Model file for the job. Use its own axes, mm. Give positions to 0.01 mm unless a question says otherwise; leave off trailing zeros. Write each loop counter-clockwise with the first axis right and the second up, starting at its lowest first coordinate (ties: lowest second). Pieces come first, ordered by that corner, then holes. Notation, with made-up numbers: (77, 78) - (93, 78) arc R17 cw to (93, 91) - close; hole circle Ø11 at (86, 54). An arc over 180 degrees is marked (long way). One line per item, written item: value. Start each with the question number.
(1) Cut at A-A, the plane y = 0. List the corners of the cut face in (x, z) (1 decimal), and give its area (3 significant figures).
(2) Cut at D-D, the plane x = 5. List the corners of the cut face in (y, z) (3 decimals), and give its area (3 significant figures).
(3) Probe L1, parallel to Y at x = 0, z = 1.2; L2, parallel to Y at x = 8, z = 1.7; L3, parallel to X at y = -14, z = 1.15. List the from-to ranges inside material, lowest first.
(4) Drop a flat-ended pin along its axis: P1, Ø1, axis at y = 10.5, z = 2, coming from the -X side. Give the stop position or say it passes through.
(5) Cut at C-C, the plane z = 1.3. List the corners of the cut face in (x, y) (1 decimal).
(6) Cut at B-B, the plane x = 0. List the corners of the cut face in (y, z) (3 decimals), and give its area (3 significant figures).
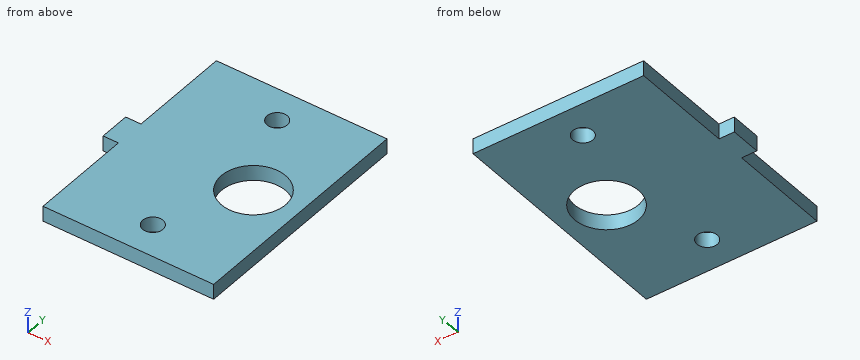
from build123d import *

# Parameters (mm, degrees)
SKETCH1_W           = 35.47213452
SKETCH1_H           = 48.789667988
BOSS_EXTRUDE1_DEPTH = 3.175
SKETCH2_R           = 2.10185
SKETCH2_R_2         = 6.6675
CUT_EXTRUDE1_DEPTH  = 31.327489716
BOSS_EXTRUDE2_DEPTH = 3.175


with BuildPart() as part:
    # Sketch1 → Boss-Extrude1 (new body)
    with BuildSketch(Plane.XY):
        Rectangle(SKETCH1_W, SKETCH1_H)
    extrude(amount=BOSS_EXTRUDE1_DEPTH)

    # Sketch2 → Cut-Extrude1 (cut, through all)
    with BuildSketch(Plane(origin=(0, 0, 0), x_dir=(-1, 0, 0), z_dir=(0, 0, -1))):
        with Locations((0, 17.5)):
            Circle(SKETCH2_R)
        with Locations((0, -17.5)):
            Circle(SKETCH2_R)
        with Locations((-8, 0)):
            Circle(SKETCH2_R_2)
    extrude(amount=-CUT_EXTRUDE1_DEPTH, mode=Mode.SUBTRACT)

    # Sketch3 → Boss-Extrude2 (add)
    with BuildSketch(Plane.ZY.offset(17.73606726)):
        Polygon((0, 0), (0, -3.175), (3.175, -3.175), (3.175, 3.175), (0, 3.175), align=None)
    extrude(amount=BOSS_EXTRUDE2_DEPTH)


solid = part.part
Answers follow:
1. outline: (-20.9, 0) - (1.3, 0) - (1.3, 3.2) - (-20.9, 3.2) - close; (14.7, 0) - (17.7, 0) - (17.7, 3.2) - (14.7, 3.2) - close
1. area: 80.4 mm²
2. outline: (-24.395, 0) - (-5.954, 0) - (-5.954, 3.175) - (-24.395, 3.175) - close; (5.954, 0) - (24.395, 0) - (24.395, 3.175) - (5.954, 3.175) - close
2. area: 117 mm²
3. L1: y = -24.39 to -19.6, -15.4 to 15.4, 19.6 to 24.39
3. L2: y = -24.39 to -6.67, 6.67 to 24.39
3. L3: x = -17.74 to 17.74
4. P1: stops at x = -17.74
5. outline: (-20.9, -3.2) - (-17.7, -3.2) - (-17.7, -24.4) - (17.7, -24.4) - (17.7, 24.4) - (-17.7, 24.4) - (-17.7, 3.2) - (-20.9, 3.2) - close; hole circle Ø4.2 at (0, -17.5); hole circle Ø4.2 at (0, 17.5); hole circle Ø13.3 at (8, 0)
6. outline: (-24.395, 0) - (-19.602, 0) - (-19.602, 3.175) - (-24.395, 3.175) - close; (-15.398, 0) - (15.398, 0) - (15.398, 3.175) - (-15.398, 3.175) - close; (19.602, 0) - (24.395, 0) - (24.395, 3.175) - (19.602, 3.175) - close
6. area: 128 mm²
